from build123d import *

# Parameters (mm, degrees)
F0_W     = 69.863096
F0_H     = 137.526572
F2_DEPTH = 76.89179
F1_R     = 9.824635
F4_DEPTH = 25.4
F5_DEPTH = 38.1


with BuildPart() as f2:
    # F0 (on Top) → F2 (new body)
    with BuildSketch(Plane.XY):
        with Locations((-34.931548, 0)):
            Rectangle(F0_W, F0_H)
        with Locations((34.931548, 0)):
            Rectangle(F0_W, F0_H)
    extrude(amount=-F2_DEPTH)

    # F1 (on Top) → F3 (revolve)
    with BuildSketch(Plane.XY):
        with Locations((54.264009, 0)):
            Circle(F1_R)
    revolve(axis=Axis((0, 0, 0), (0, -1, 0)))

    # F0 (on Top) → F4 (join)
    with BuildSketch(Plane.XY):
        with Locations((34.931548, 0)):
            Rectangle(F0_W, F0_H)
    extrude(amount=-F4_DEPTH)

    # F0 (on Top) → F5 (cut)
    with BuildSketch(Plane.XY):
        with Locations((34.931548, 0)):
            Rectangle(F0_W, F0_H)
    extrude(amount=-F5_DEPTH, mode=Mode.SUBTRACT)


solid = f2.part
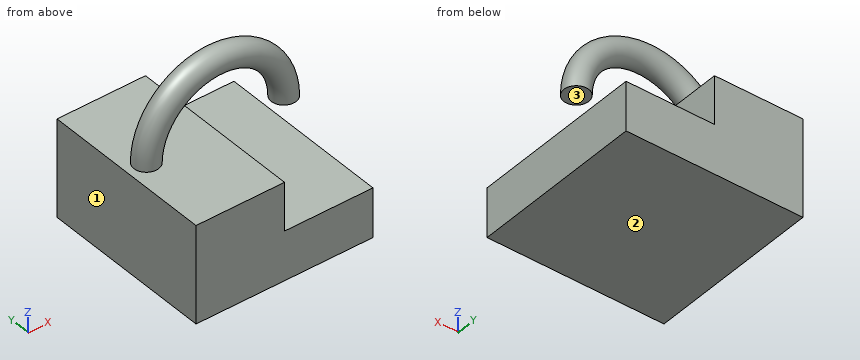
Geometry: final body of the model. Coordinates: model frame, mm. Face numbers are marked on the shaded views. Give positions to 0.01 mm unless a question says otherwise; leave off trailing zeros. Loops run counter-clockwise (first coordinate to the right, second up) from the corner with the lowest first, then second, coordinate; pieces in that order, holes last. Notation, with made-up numbers: (20, 88) - (60, 88) arc R24 ccw to (60, 126) - close; hole circle Ø10 at (66, -11). An arc over 180 degrees is marked (long way). Answer as CSV lines item,"result". Start each with the question number.
1. Section B-B, the plane z = -6. Return loops of the section in (x, y), plus the area to 3 significant figures.
2. Section A-A, the plane y = 56. Return loops of the section in (x, z), plus the area to 3 significant figures.
3. Draft query along Z for the marked faces 1, 2 and 3. Return one class per face: released by +Z, released by -Z, zero draft, split by the parting line, or undercut.
4. Section C-C, the plane y = 4. Return loops of the section in (x, z) (1 decimal).
5. Ray query, L1, parallel to Z at x = 34, y = -18.5; L2, parallel to Z at x = -5.5, y = -24; L3, parallel to X at y = 48, z = -28. Return the intervals inside material, ascending.
6. Pin query (flat end, axial travel): P1, Ø12, axis at x = -27, z = 37.5, coming from the +Y side; P2, Ø21, axis at x = 38, y = 25, coming from the +Z side; P3, Ø19, axis at y = -10, z = -17.5, coming from the +X side. Return the tip coordinate at first contact, or that it passes through.
Answers:
1,outline,"(-69.86, -68.76) - (0, -68.76) - (0, 68.76) - (-69.86, 68.76) - close"
1,area,"9,610 mm2"
2,outline,"(-69.86, -76.89) - (69.86, -76.89) - (69.86, -38.1) - (0, -38.1) - (0, 0) - (-69.86, 0) - close"
2,area,"8,080 mm2"
3,face 1,"zero draft"
3,face 2,"released by -Z"
3,face 3,"undercut"
4,outline,"(-69.9, -76.9) - (69.9, -76.9) - (69.9, -38.1) - (0, -38.1) - (0, 0) - (-45.3, 0) arc R45.3 cw to (45.3, 0) - (63.2, 0) arc R63.2 ccw to (-63.2, 0) - (-69.9, 0) - close"
5,L1,"z = -76.89 to -38.1"
5,L2,"z = -76.89 to 0"
5,L3,"x = -69.86 to 0"
6,P1,"stops at y = 9.61"
6,P2,"stops at z = -38.1"
6,P3,"stops at x = 0"
